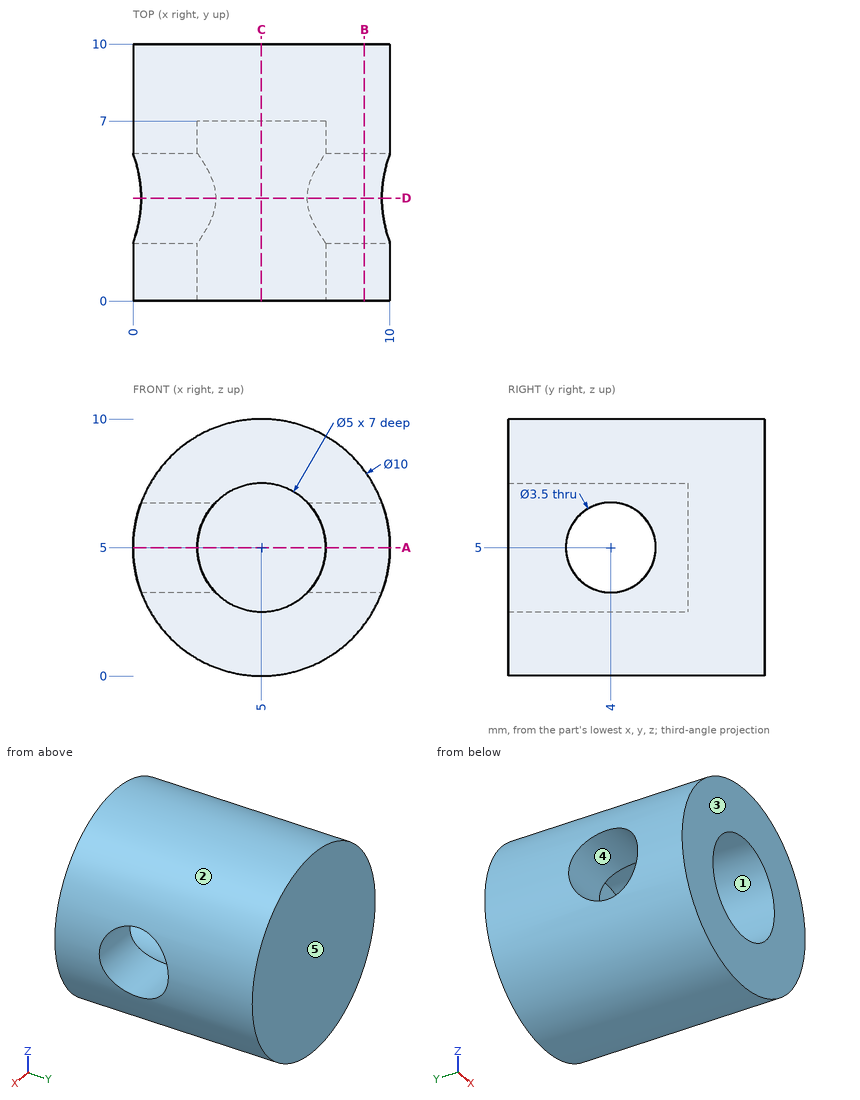
Geometry check sheet. Reference: drawing and pictorial views, mm from the part's lowest x, y, z. A direction names the side the tool comes from. Coordinates: 2 decimals unless noted, no trailing zeros. Loops run counter-clockwise (first coordinate to the right, second up) from the corner with the lowest first, then second, coordinate; pieces in that order, holes last. Notation, with made-up numbers: (1.25, 37) -> (27.25, 37) arc R17 ccw to (27.25, 42) -> close; hole circle Ø6 at (36.5, 68). An arc over 180 degrees is marked (long way). Put each result on its own line as item: value.
1) Tool access check on the marked faces 1 and 2. Record the directions out of +Z, -Z, +X, -X, +Y, -Y that give a thin tool (end or side, any length) a straight path to the whole face; none if there is none.
Result set:
face 1: -Y
face 2: +Y, -Y
2) Gauge pin test, flat ends, axial feed: pin 1 Ø5.5 at (y, z) = (4, 5) entering from +X; pin 2 Ø4 at (y, z) = (2.5, 8) entering from -X. Record the tip position at first contact, or that the pin passes through.
Result set:
pin 1: stops at x = 10
pin 2: stops at x = 0.1
3) Cross-section at D-D on y = 4. Record the boundary of the cut face in (x, z).
Result set:
outline: (0.32, 3.25) arc R5 ccw to (9.68, 3.25) -> (6.79, 3.25) arc R2.5 cw to (3.21, 3.25) -> close; (0.32, 6.75) -> (3.21, 6.75) arc R2.5 cw to (6.79, 6.75) -> (9.68, 6.75) arc R5 ccw to start
4) Release check for a two-part mould opening along Y. For the marked faces 3, 4 and 5 record: released by +Y, released by -Y, zero draft, split by the parting line, or undercut.
Result set:
face 3: released by -Y
face 4: undercut
face 5: released by +Y
5) Cross-section at B-B on x = 9. Record the boundary of the cut face in (y, z).
Result set:
outline: (0, 2) -> (10, 2) -> (10, 8) -> (0, 8) -> close; hole circle Ø3.5 at (4, 5)
6) Cross-section at C-C on x = 5. Record the boundary of the cut face in (y, z).
Result set:
outline: (0, 0) -> (10, 0) -> (10, 10) -> (0, 10) -> (0, 7.5) -> (7, 7.5) -> (7, 2.5) -> (0, 2.5) -> close
7) Cross-section at A-A on z = 5. Record the boundary of the cut face in (x, y), plus the area to 3 significant figures.
Result set:
outline: (0, 0) -> (2.5, 0) -> (2.5, 2.25) -> (0, 2.25) -> close; (0, 5.75) -> (2.5, 5.75) -> (2.5, 7) -> (7.5, 7) -> (7.5, 5.75) -> (10, 5.75) -> (10, 10) -> (0, 10) -> close; (7.5, 0) -> (10, 0) -> (10, 2.25) -> (7.5, 2.25) -> close
area: 47.5 mm^2
8) Thickness scan on line 1 (Z direction, x = 5, y = 5.5); line 2 (Z direction, x = 6, y = 6.5); line 3 (X direction, y = 6, z = 7). Record the ranges inside material, lowest first.
Result set:
line 1: z = 0 to 2.5, 7.5 to 10
line 2: z = 0.1 to 2.71, 7.29 to 9.9
line 3: x = 0.42 to 3.5, 6.5 to 9.58
